Here's how the part is built. I have some questions about the finished solid (model axes, mm). A direction names the side the tool comes from. Round coordinates to 2 decimals unless told otherwise and drop trailing zeros. Write each loop counter-clockwise with the first axis right and the second up, starting at its lowest first coordinate (ties: lowest second). Pieces come first, ordered by that corner, then holes. Notation, with made-up numbers: M 40,9 L 45,9 A20 ccw 45,35 Z; hole C 61,8 d6. An arc over 180 degrees is marked long. Write item = value, one per line. Start each with the question number.
(1) I want a section at D-D (x = 17). Give the number of separate pieces and of enclosed holes in the cut face, and give its area (3 significant figures).
(2) I want a section at A-A (z = 8.75). List the corners of the cut face in (x, y) for me.
(3) I need wall thicknesses on line 1 along X through (y, z) = (-26.5, -8); line 2 along Z through (x, y) = (-32, 53.5); line 3 along Y through (x, z) = (16.5, -2). Which ranges of each line are inside material? Lowest first, please.
(4) On a 3-axis mill with a long thin cutter (end or side, diameter ignored), from which of +Z, -Z, +X, -X, +Y, -Y can I reach the whole of each face in a straight line? I mean faces 4 (the cylindrical face through (33.59, 1.95, 2.67)), 5 (the flat face through (-40.08, -23.58, 3.45)), 6 (the flat face through (26.847, 43, 3)), 7 (the flat face through (-33, 1, -10.3)). Say none if no direction works.
(5) I want a section at B-B (y = 55.5). List the corners of the cut face in (x, z) for me.
(6) I want a section at C-C (z = -3). List the corners of the cut face in (x, y) for me, and give its area (3 significant figures).
(7) If we mould it in two halves opening along X, with no side actions, what happens to faces 1 (the flat face through (-26.847, 42, 3)), 2 (the flat face through (-1, 1, -13)), 3 (the cylindrical face through (-19.9, -11.9, 5.1))? For each: released by +X, released by -X, zero draft, split by the parting line, or undercut.
(8) Will these pins go through, and if not, where does the flat tip stop? pin 1 Ø12 at (y, z) = (-49, -2) entering from -X; pin 2 Ø12.5 at (x, y) = (45.5, -5.5) entering from -Z; pin 3 Ø10 at (x, y) = (-24, -11) entering from +Z.
```python
from build123d import *

# Parameters (mm, degrees)
RESSALTO_EXTRUS_O1_DEPTH = 7
RESSALTO_EXTRUS_O2_DEPTH = 5
RESSALTO_EXTRUS_O3_DEPTH = 13
CORTE_EXTRUS_O1_START    = -131
CORTE_EXTRUS_O1_DEPTH    = 131
CORTE_EXTRUS_O2_DEPTH    = 60
CORTE_EXTRUS_O3_DEPTH    = 58
CORTE_EXTRUS_O4_DEPTH    = 53
CORTE_EXTRUS_O5_DEPTH    = 3.4
ESBO_O13_W               = 62.4
ESBO_O13_H               = 52.25073341
ESBO_O13_H_2             = 58.74926659
CORTE_EXTRUS_O6_DEPTH    = 3.4


# Read off the part's stored shape, not the designer's step: Corte-extrus_o1
with BuildPart() as part:
    # Esbo_o1 → Ressalto-extrus_o1 (new body)
    with BuildSketch(Plane.XY):
        with BuildLine():
            Line((-26.846787517, 46.5), (26.846787517, 46.5))
            Line((26.846787517, 46.5), (26.846787517, 38.5))
            ThreePointArc((26.846787517, 38.5), (16.603731122, 25.147195766), (9.603000417, 9.843361122))
            ThreePointArc((9.603000417, 9.843361122), (10.024733627, 5.787782658), (13.326100999, 3.394761752))
            ThreePointArc((13.326100999, 3.394761752), (30.079975929, 1.805655066), (46.765371804, 4))
            Line((46.765371804, 4), (53.693575035, 0))
            Line((53.693575035, 0), (26.846787517, -46.5))
            Line((26.846787517, -46.5), (19.918584287, -42.5))
            ThreePointArc((19.918584287, -42.5), (13.476244807, -26.952850832), (3.723100582, -13.238122875))
            ThreePointArc((3.723100582, -13.238122875), (0, -11.575565317), (-3.723100582, -13.238122875))
            ThreePointArc((-3.723100582, -13.238122875), (-13.476244807, -26.952850832), (-19.918584287, -42.5))
            Line((-19.918584287, -42.5), (-26.846787517, -46.5))
            Line((-26.846787517, -46.5), (-53.693575035, 0))
            Line((-53.693575035, 0), (-46.765371804, 4))
            ThreePointArc((-46.765371804, 4), (-30.079975929, 1.805655066), (-13.326100999, 3.394761752))
            ThreePointArc((-13.326100999, 3.394761752), (-10.024733627, 5.787782658), (-9.603000417, 9.843361122))
            ThreePointArc((-9.603000417, 9.843361122), (-16.603731122, 25.147195766), (-26.846787517, 38.5))
            Line((-26.846787517, 38.5), (-26.846787517, 46.5))
        make_face()
    extrude(amount=RESSALTO_EXTRUS_O1_DEPTH)

    # Esbo_o2 → Ressalto-extrus_o2 (add)
    with BuildSketch(Plane.XY.offset(7)):
        Polygon((37.239092363, -21.5), (44.739092363, -8.509618943), (42.574028853, -7.259618943), (27.574028853, -33.240381057), (29.739092363, -34.490381057), align=None)
        Polygon((0, 43), (-15, 43), (-15, 40.5), (15, 40.5), (15, 43), align=None)
        Polygon((-37.239092363, -21.5), (-29.739092363, -34.490381057), (-27.574028853, -33.240381057), (-42.574028853, -7.259618943), (-44.739092363, -8.509618943), align=None)
    extrude(amount=RESSALTO_EXTRUS_O2_DEPTH)

    # Esbo_o3 → Ressalto-extrus_o3 (add)
    with BuildSketch(Plane(origin=(0, 0, 0), x_dir=(-1, 0, 0), z_dir=(0, 0, -1))):
        with BuildLine():
            Line((38, 63.25073341), (38, -63.25073341))
            ThreePointArc((38, -63.25073341), (36.828427125, -66.079160535), (34, -67.25073341))
            Line((34, -67.25073341), (-34, -67.25073341))
            ThreePointArc((-34, -67.25073341), (-36.828427125, -66.079160535), (-38, -63.25073341))
            Line((-38, -63.25073341), (-38, 63.25073341))
            ThreePointArc((-38, 63.25073341), (-36.828427125, 66.079160535), (-34, 67.25073341))
            Line((-34, 67.25073341), (34, 67.25073341))
            ThreePointArc((34, 67.25073341), (36.828427125, 66.079160535), (38, 63.25073341))
        make_face()
    extrude(amount=RESSALTO_EXTRUS_O3_DEPTH)

    # Corte-extrus_o1 outline → Corte-extrus_o1 (cut)
    with BuildSketch(Plane(origin=(0, 67.25073341, 0), x_dir=(1, 0, 0), z_dir=(0, 1, 0)).offset(CORTE_EXTRUS_O1_START)):
        Polygon((31.2, 11.3), (-31.2, 11.3), (-31.2, 10.3), (-34, 10.3), (-34, 1), (34, 1), (34, 10.3), (31.2, 10.3), align=None)
    extrude(amount=CORTE_EXTRUS_O1_DEPTH, mode=Mode.SUBTRACT)

    # Esbo_o6 → Corte-extrus_o2 (cut)
    with BuildSketch(Plane.ZY.offset(26.846787517)):
        with BuildLine():
            Line((18.516337651, 34.944688344), (7, 34.944688344))
            ThreePointArc((7, 34.944688344), (4.663173788, 19.541492285), (3.576332881, 4))
            Line((3.576332881, 4), (21.222643852, 4))
            Line((21.222643852, 4), (18.516337651, 34.944688344))
        make_face()
    extrude(amount=-CORTE_EXTRUS_O2_DEPTH, mode=Mode.SUBTRACT)

    # Esbo_o8 → Corte-extrus_o3 (cut)
    with BuildSketch(Plane(origin=(13.423393759, -23.25, 0), x_dir=(0.8660254037844386, 0.5000000000000003, 0), z_dir=(0.5000000000000003, -0.8660254037844386, 0))):
        with BuildLine():
            Line((-34.944688344, 18.516337651), (-34.944688344, 7))
            ThreePointArc((-34.944688344, 7), (-19.541492285, 4.663173788), (-4, 3.576332881))
            Line((-4, 3.576332881), (-4, 21.222643852))
            Line((-4, 21.222643852), (-34.944688344, 18.516337651))
        make_face()
    extrude(amount=-CORTE_EXTRUS_O3_DEPTH, mode=Mode.SUBTRACT)

    # Esbo_o10 → Corte-extrus_o4 (cut)
    with BuildSketch(Plane(origin=(13.423393759, 23.25, 0), x_dir=(0.8660254037845888, -0.4999999999997399, 0), z_dir=(0.49999999999973993, 0.8660254037845889, 0))):
        with BuildLine():
            Line((34.944688344, -18.516337651), (34.944688344, -7))
            ThreePointArc((34.944688344, -7), (19.541492285, -4.663173788), (4, -3.576332881))
            Line((4, -3.576332881), (4, -21.222643852))
            Line((4, -21.222643852), (34.944688344, -18.516337651))
        make_face()
    extrude(amount=-CORTE_EXTRUS_O4_DEPTH, mode=Mode.SUBTRACT)

    # Esbo_o11 → Corte-extrus_o5 (cut)
    with BuildSketch(Plane.XY.offset(7)):
        Polygon((-6.92820323, 4), (6.92820323, 4), (0, -8), align=None)
    extrude(amount=-CORTE_EXTRUS_O5_DEPTH, mode=Mode.SUBTRACT)

    # Esbo_o13 → Corte-extrus_o6 (cut)
    with BuildSketch(Plane(origin=(0, 0, -13), x_dir=(-1, 0, 0), z_dir=(0, 0, -1))):
        with Locations((0, 31.125366705)):
            Rectangle(ESBO_O13_W, ESBO_O13_H)
        with Locations((0, -34.374633295)):
            Rectangle(ESBO_O13_W, ESBO_O13_H_2)
    extrude(amount=-CORTE_EXTRUS_O6_DEPTH, mode=Mode.SUBTRACT)


solid = part.part
```
Returned:
q1.separate_pieces = 3
q1.enclosed_holes = 0
q1.area = 536 mm²
q2.outline = M -44.74,-8.51 L -29.74,-34.49 L -27.57,-33.24 L -42.57,-7.26 Z; M -15,40.5 L 15,40.5 L 15,43 L -15,43 Z; M 27.57,-33.24 L 29.74,-34.49 L 44.74,-8.51 L 42.57,-7.26 Z
q3.line_1 = -38 to -34, 34 to 38
q3.line_2 = -13 to -10.3, -1 to 0
q3.line_3 = -67.25 to -63.75
q4.face_4 = +Z
q4.face_5 = +Z, -X, -Y
q4.face_6 = +Z, +X, +Y
q4.face_7 = +Y
q5.outline = M -38,-13 L -31.2,-13 L -31.2,-10.3 L -34,-10.3 L -34,-1 L 34,-1 L 34,-10.3 L 31.2,-10.3 L 31.2,-13 L 38,-13 L 38,0 L -38,0 Z
q6.outline = M -38,-63.25 A4 ccw -34,-67.25 L 34,-67.25 A4 ccw 38,-63.25 L 38,63.25 A4 ccw 34,67.25 L 34,-63.75 L -34,-63.75 L -34,67.25 A4 ccw -38,63.25 Z
q6.area = 1,300 mm²
q7.face_1 = released by -X
q7.face_2 = zero draft
q7.face_3 = undercut
q8.pin_1 = -38
q8.pin_2 = 0
q8.pin_3 = 6.33
